The listing builds one solid part. Answer for the finished solid, in the listing's coordinates (mm). A direction names the side the tool comes from. Give positions to 0.01 mm unless a question says otherwise; leave off trailing zeros. Loops run counter-clockwise (first coordinate to the right, second up) from the corner with the lowest first, then second, coordinate; pieces in that order, holes last. Notation, with made-up numbers: M 77.25,-17 L 125.25,-17 A22 ccw 125.25,21 Z; hole C -4,16 d10. An arc over 180 degrees is marked long. Return JSON: item names as keys, results as strings.
from build123d import *

# Parameters (mm, degrees)
SKETCH1_W           = 11000
SKETCH1_H           = 2000
BOSS_EXTRUDE1_DEPTH = 1250
SKETCH2_R           = 815
CUT_EXTRUDE2_DEPTH  = 410
SKETCH23_R          = 312.5
CUT_EXTRUDE3_DEPTH  = 11251
SKETCH24_R          = 130
CUT_EXTRUDE4_DEPTH  = 11251
SKETCH25_R          = 130
CUT_EXTRUDE5_DEPTH  = 11251
SCALE1_SCALE        = 0.025


with BuildPart() as part:
    # Sketch1 → Boss-Extrude1 (new body)
    with BuildSketch(Plane.XY):
        with Locations((5500, 1000)):
            Rectangle(SKETCH1_W, SKETCH1_H)
    extrude(amount=-BOSS_EXTRUDE1_DEPTH)

    # Sketch2 → Cut-Extrude2 (cut)
    with BuildSketch(Plane.XY):
        with Locations((2200, 1000)):
            Circle(SKETCH2_R)
        with Locations((8800, 1000)):
            Circle(SKETCH2_R)
    extrude(amount=-CUT_EXTRUDE2_DEPTH, mode=Mode.SUBTRACT)

    # Sketch23 → Cut-Extrude3 (cut, through all)
    with BuildSketch(Plane.XY):
        with Locations((2200, 1000)):
            Circle(SKETCH23_R)
        with Locations((8800, 1000)):
            Circle(SKETCH23_R)
    extrude(amount=-CUT_EXTRUDE3_DEPTH, mode=Mode.SUBTRACT)

    # Sketch24 → Cut-Extrude4 (cut, through all)
    with BuildSketch(Plane.XY):
        with Locations((2200, 435)):
            Circle(SKETCH24_R)
        with Locations((1635, 1000)):
            Circle(SKETCH24_R)
        with Locations((2200, 1565)):
            Circle(SKETCH24_R)
        with Locations((2765, 1000)):
            Circle(SKETCH24_R)
    extrude(amount=-CUT_EXTRUDE4_DEPTH, mode=Mode.SUBTRACT)

    # Sketch25 → Cut-Extrude5 (cut, through all)
    with BuildSketch(Plane.XY):
        with Locations((8800, 435)):
            Circle(SKETCH25_R)
        with Locations((8235, 1000)):
            Circle(SKETCH25_R)
        with Locations((8800, 1565)):
            Circle(SKETCH25_R)
        with Locations((9365, 1000)):
            Circle(SKETCH25_R)
    extrude(amount=-CUT_EXTRUDE5_DEPTH, mode=Mode.SUBTRACT)


with BuildPart() as part_1:
    # Scale1: scaled about (5500, 1000, -646.66686697)
    add(part.part.scale(SCALE1_SCALE).moved(Location((5362.5, 975, -630.500195296))))


solid = part_1.part
(1) Straight lines are drawn through the part: line 1 along Y through (x, z) = (5582.5, -645.5) (1 decimal); line 2 along Y through (x, z) = (5417, -653); line 3 along X through (y, z) = (1003.5, -636.5). For each, find the intervals that lie inside material, in ascending order.
Values follow:
{"line 1": "975 to 982.6, 989.1 to 992.2, 1007.8 to 1010.9, 1017.4 to 1025", "line 2": "975 to 982.66, 989.09 to 992.2, 1007.8 to 1010.91, 1017.34 to 1025", "line 3": "5362.5 to 5397.43, 5437.57 to 5562.43, 5602.57 to 5637.5"}
(2) A tool of negligible diameter and unlimited length cuts with its end or side. For faces 4 (the cylindrical face through (5580.105, 988.072, -651.103)), 5 (the cylindrical face through (5562.145, 1000.896, -635.553)), from which of +Z, -Z, +X, -X, +Y, -Y can it reach the whole face along a straight path? Write none if from no direction.
Values follow:
{"face 4": "+Z, -Z", "face 5": "+Z"}
(3) The part is cut by section A-A (x = 5417.5). Determine the outline of the cut face in (y, z) (1 decimal), and give its area (3 significant figures).
Values follow:
{"outline": "M 975,-661.8 L 982.6,-661.8 L 982.6,-640.8 L 979.6,-640.8 L 979.6,-630.5 L 975,-630.5 Z; M 989.1,-661.8 L 992.2,-661.8 L 992.2,-640.8 L 989.1,-640.8 Z; M 1007.8,-661.8 L 1010.9,-661.8 L 1010.9,-640.8 L 1007.8,-640.8 Z; M 1017.4,-661.8 L 1025,-661.8 L 1025,-630.5 L 1020.4,-630.5 L 1020.4,-640.8 L 1017.4,-640.8 Z", "area": "544 mm²"}
(4) Determine the mould class of faces 1 (the flat face through (5362.5, 1000, -646)), 2 (the flat face through (5582, 991, -640.75)), 3 (the flat face through (5637.5, 1000, -646)) for opening direction X: released by +X, released by -X, zero draft, split by the parting line, or undercut.
Values follow:
{"face 1": "released by -X", "face 2": "undercut", "face 3": "released by +X"}
(5) The part is cut by section B-B (z = -652.5). Give the number of separate pieces and of enclosed holes in the cut face, and give its area (3 significant figures).
Values follow:
{"separate pieces": "1", "enclosed holes": "10", "area": "13,100 mm²"}
(6) Given pin 1 (18 mm diameter, centred on x = 5582.5, y = 1000, fed in from -Z); pin 2 (4 mm diameter, centred on x = 5582.5, y = 1014.125, fed in from +Z); pin 3 (10.5 mm diameter, centred on x = 5582.5, y = 985.875, fed in from +Z), each flat-ended and moving along its own axis, determine where each tip first touches the part or whether it passes through.
Values follow:
{"pin 1": "z = -661.75", "pin 2": "through", "pin 3": "z = -640.75"}
